from build123d import *

# Parameters (mm, degrees)
IZIM1_W = 1
IZIM1_H = 0.5


with BuildPart() as part:
    # Süpür1: sweep along a path in Çizim2
    with BuildLine(Plane(origin=(0, 0, 0), x_dir=(0, 0, -1), z_dir=(1, 0, 0))) as s_p_r1_path:
        Line((0, 0), (20.925351885, 5.491949727))
        ThreePointArc((20.925351885, 5.491949727), (25.014077523, 5.844705367), (28.985134799, 4.808936092))
        Line((28.985134799, 4.808936092), (37.108981933, 1.124891018))
        ThreePointArc((37.108981933, 1.124891018), (46.985809894, 7.054511358), (37.942195071, 14.190697936))
        Line((37.942195071, 14.190697936), (30.12359745, 11.785993841))
        ThreePointArc((30.12359745, 11.785993841), (25.171390105, 10.89789359), (20.150614238, 11.22175983))
        Line((20.150614238, 11.22175983), (0, 15))
    # Çizim1 → Süpür1 (sweep)
    with BuildSketch(Plane.XY):
        Rectangle(IZIM1_W, IZIM1_H)
    sweep(path=s_p_r1_path.line)


solid = part.part
For this review, take the finished solid that the model builds, in its own axes (mm). A direction names the side the tool comes from. Round coordinates to 2 decimals unless told otherwise and drop trailing zeros. Loops run counter-clockwise (first coordinate to the right, second up) from the corner with the lowest first, then second, coordinate; pieces in that order, holes last. Notation, with made-up numbers: (6.25, 78.25) - (60.25, 78.25) arc R24 ccw to (60.25, 101.25) - close; hole circle Ø6 at (24.25, 45). An arc over 180 degrees is marked (long way). Use one line per item in the form item = value.
1) We need section D-D on z = -11.5. Write out the cut boundary in (x, y).
Solutions:
outline = (-0.5, 2.77) - (0.5, 2.77) - (0.5, 3.27) - (-0.5, 3.27) - close; (-0.5, 12.6) - (0.5, 12.6) - (0.5, 13.09) - (-0.5, 13.09) - close
2) We need section B-B on x = 0.1. Write out the cut boundary in (y, z).
Solutions:
outline = (-0.25, 0) - (5.24, -20.93) arc R11.84 cw to (4.61, -28.83) - (0.93, -36.95) arc R7.24 ccw (long way) to (14.44, -37.93) - (12.04, -30.11) arc R20.61 cw to (11.45, -20.26) - (15.23, -0.11) - (14.77, 0.11) - (11, -20.04) arc R21.09 ccw to (11.54, -30.13) - (13.94, -37.95) arc R6.76 cw (long way) to (1.32, -37.27) - (5, -29.14) arc R12.33 ccw to (5.74, -20.93) - (0.25, 0) - close
3) We need section A-A on z = -40. Write out the cut boundary in (x, y).
Solutions:
outline = (-0.5, 0.26) - (0.5, 0.26) - (0.5, 0.74) - (-0.5, 0.74) - close; (-0.5, 14.26) - (0.5, 14.26) - (0.5, 14.74) - (-0.5, 14.74) - close
4) Tool access review of faces 4 (the face through (0.007, 3.034, -10.609)), 5 (the face through (-0.007, 13.363, -10.041)), 6 (the face through (-0.5, 5.8, -25.4)), 7 (the face through (0.007, 3.135, -33.262)), 8 (the face through (-0.007, 2.747, -32.946)): name each direction out of +Z, -Z, +X, -X, +Y, -Y from which nothing blocks a thin tool from reaching the whole face with its end or side.
Solutions:
face_4 = +Z, +X, -X
face_5 = +X, -X, +Y
face_6 = +Z, -Z, -X, +Y, -Y
face_7 = +X, -X
face_8 = +X, -X, -Y
5) Mouldability with a two-part tool opening along Z and no side actions: class faces 1 (the face through (0.5, 5.73, -25.43)), 2 (the face through (0.01, 12.91, -9.83)), 3 (the face through (-0.007, 6.951, -46.736)) as pulls with the +Z half, pulls with the -Z half, needs draft (parallel to the pull), parting line crosses it, or undercut.
Solutions:
face_1 = needs draft
face_2 = pulls with the +Z half
face_3 = undercut
6) Wall thickness on probe 1 along Y at (x, z) = (0, -24); probe 2 along Y at (x, z) = (0.35, -40); probe 3 along Z at (x, y) = (-0.15, 7.5): over which ranges is each line inside the solid? List them lowest first.
Solutions:
probe_1 = 5.65 to 6.13, 10.62 to 11.11
probe_2 = 0.26 to 0.74, 14.26 to 14.74
probe_3 = -47.24 to -46.76
7) We need section C-C on y = 2.5. Write out the cut boundary in (x, z).
Solutions:
outline = (-0.5, -45.24) - (0.5, -45.24) - (0.5, -44.55) - (-0.5, -44.55) - close; (-0.5, -34.66) - (0.5, -34.66) - (0.5, -33.49) - (-0.5, -33.49) - close; (-0.5, -10.48) - (0.5, -10.48) - (0.5, -8.57) - (-0.5, -8.57) - close
